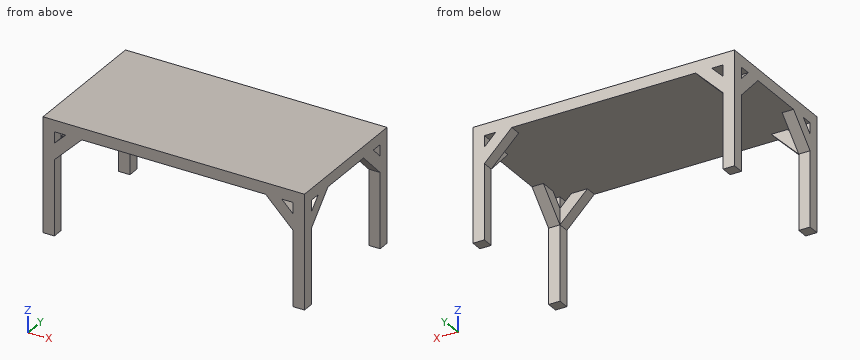
```python
from build123d import *

# Parameters (mm, degrees)
F0_W     = 575
F0_H     = 300
F1_DEPTH = 50
F2_W     = 50
F2_H     = 50
F3_DEPTH = 450
F5_DEPTH = 50
F7_DEPTH = 50


with BuildPart() as f1:
    # F0 (on Top) → F1 (new body)
    with BuildSketch(Plane.XY):
        with Locations((287.5, -150)):
            Rectangle(F0_W, F0_H)
    extrude(amount=-F1_DEPTH)

    # F2 (on face) → F3 (join)
    with BuildSketch(Plane(origin=(0, 0, -50), x_dir=(1, 0, 0), z_dir=(0, 0, -1))):
        with Locations((550, 275)):
            Rectangle(F2_W, F2_H)
    extrude(amount=F3_DEPTH)

    # F4 (on face) → F5 (join, through all)
    with BuildSketch(Plane.XZ.offset(300)):
        Polygon((525, -170.710678), (525, -100), (475, -50), (404.289322, -50), align=None)
    extrude(amount=-F5_DEPTH)

    # F6 (on face) → F7 (join, through all)
    with BuildSketch(Plane.YZ.offset(575)):
        Polygon((-200, -50), (-250, -100), (-250, -170.710678), (-129.289322, -50), align=None)
    extrude(amount=-F7_DEPTH)

    # F8: F1 across plane


with BuildPart() as f1_1:
    add(f1.part)
    add(f1.part.mirror(Plane.YZ))

    # F9: F1 across plane


with BuildPart() as f1_2:
    add(f1_1.part)
    add(f1_1.part.mirror(Plane.XZ))


solid = f1_2.part
```
Here's how the part is built. I have some questions about the finished solid (model axes, mm). Round coordinates to 2 decimals unless told otherwise and drop trailing zeros. Order: outer loops, then holes, each group sorted by start corner. A loop starts at its lowest first (then second) coordinate and runs counter-clockwise, first axis right, second up. Notation, with made-up numbers: M 86.5,89.25 L 105.5,89.25 A23 ccw 105.5,113.25 Z; hole C 58,76 d9. An arc over 180 degrees is marked long. Answer in a Markdown table with one row per item.
Item 1: Imagine slicing it at A-A, the plane z = -210. Write out the boundary of the cut face in (x, y).
A:
| item | result |
|---|---|
| outline | M -575,-300 L -525,-300 L -525,-250 L -575,-250 Z; M -575,250 L -525,250 L -525,300 L -575,300 Z; M 525,-300 L 575,-300 L 575,-250 L 525,-250 Z; M 525,250 L 575,250 L 575,300 L 525,300 Z |
Item 2: I'm going to push a flat-ended pin straight in: pin 1 (1 mm diameter, centred on x = 343.5, y = 141, fed in from -Z). Where does the tip first touch, or does it pass through?
A:
| item | result |
|---|---|
| pin 1 | stops at z = -50 |
Item 3: Imagine slicing it at D-D, the plane z = -88. State how many separate pieces and enclosed holes the cut face has, and give its area (3 significant figures).
A:
| item | result |
|---|---|
| separate pieces | 12 |
| enclosed holes | 0 |
| area | 38,300 mm2 |
Item 4: If I drill on L1, parallel to Z at x = 526, y = 51.5; L2, parallel to X at y = -255, z = -479, over which ranges is the centre line in solid material (lowest first)? Write a range as from..to.
A:
| item | result |
|---|---|
| L1 | z = -50..0 |
| L2 | x = -575..-525, 525..575 |
Item 5: Imagine slicing it at B-B, the plane y = -215. Write out the boundary of the cut face in (x, z), and give its area (3 significant figures).
A:
| item | result |
|---|---|
| outline | M -575,-135.71 L -525,-135.71 L -525,-65 L -575,-65 Z; M -575,-50 L 575,-50 L 575,0 L -575,0 Z; M 525,-135.71 L 575,-135.71 L 575,-65 L 525,-65 Z |
| area | 64,600 mm2 |
Item 6: Imagine slicing it at C-C, the plane x = 264. Write out the boundary of the cut face in (y, z).
A:
| item | result |
|---|---|
| outline | M -300,-50 L 300,-50 L 300,0 L -300,0 Z |
